from build123d import *

# Parameters (mm, degrees)
SKETCH1_R             = 9.5
SKETCH1_R_2           = 7.85
BOSS_EXTRUDE1_DEPTH   = 48
BOSS_EXTRUDE1_2_DEPTH = 48
SKETCH29_R            = 1.5
BOSS_EXTRUDE18_DEPTH  = 3
SKETCH36_R            = 1.7
BOSS_EXTRUDE26_DEPTH  = 38
SKETCH14_R            = 4.125
BOSS_EXTRUDE27_DEPTH  = 4
SKETCH34_R            = 4.2
CUT_EXTRUDE17_DEPTH   = 4.5
SKETCH38_R            = 2.15
CUT_EXTRUDE18_DEPTH   = 18.5
BOSS_EXTRUDE43_DEPTH  = 42.2
SKETCH7_R             = 1.7
BOSS_EXTRUDE44_DEPTH  = 2.8
BOSS_EXTRUDE42_START  = 25
BOSS_EXTRUDE42_DEPTH  = 6.5
BOSS_EXTRUDE45_DEPTH  = 10
SKETCH47_R            = 4
SKETCH47_R_2          = 1.5
BOSS_EXTRUDE40_DEPTH  = 1.4
CUT_EXTRUDE19_START   = -3.5
SKETCH20_R            = 1.5
SKETCH20_R_2          = 12.5
CUT_EXTRUDE19_DEPTH   = 3.5
SKETCH43_R            = 3.6
CUT_EXTRUDE22_DEPTH   = 3.5
BOSS_EXTRUDE38_DEPTH  = 4
SKETCH52_W            = 1
SKETCH52_H            = 10
BOSS_EXTRUDE36_DEPTH  = 1
SKETCH53_R            = 1.5
CUT_EXTRUDE29_DEPTH   = 4
CUT_EXTRUDE30_START   = -0.2
CUT_EXTRUDE30_DEPTH   = 0.2
CUT_EXTRUDE33_DEPTH   = 25
CUT_EXTRUDE32_DEPTH   = 8


with BuildPart() as part:
    # Sketch1 → Boss-Extrude1 (new body)
    with BuildSketch(Plane.XY):
        Circle(SKETCH1_R)
        Circle(SKETCH1_R_2, mode=Mode.SUBTRACT)
    extrude(amount=BOSS_EXTRUDE1_DEPTH)



with BuildPart() as body_2:
    # Sketch1 → Boss-Extrude1 2 (new body)
    with BuildSketch(Plane.XY):
        with Locations((52.4, 0)):
            Circle(SKETCH1_R)
        with Locations((52.4, 0)):
            Circle(SKETCH1_R_2, mode=Mode.SUBTRACT)
    extrude(amount=BOSS_EXTRUDE1_2_DEPTH)


with BuildPart() as part_1:
    add(part.part)

    add(body_2.part)  # Boss-Extrude18 merges body 2
    # Sketch29 → Boss-Extrude18 (add)
    with BuildSketch(Plane(origin=(0, 0, 0), x_dir=(-1, 0, 0), z_dir=(0, 0, -1))):
        with BuildLine():
            Line((-52.4, 9.5), (0, 9.5))
            ThreePointArc((0, 9.5), (-6.717514421, -6.717514421), (9.5, 0))
            Line((9.5, 0), (9.5, -54.1))
            ThreePointArc((9.5, -54.1), (6.717514421, -60.817514421), (0, -63.6))
            Line((0, -63.6), (-52.4, -63.6))
            ThreePointArc((-52.4, -63.6), (-59.117514421, -60.817514421), (-61.9, -54.1))
            Line((-61.9, -54.1), (-61.9, 0))
            ThreePointArc((-61.9, 0), (-53.919565268, -9.377682091), (-43.386121811, -3))
            ThreePointArc((-43.386121811, -3), (-43.093228593, -3.707106781), (-42.386121811, -4))
            Line((-42.386121811, -4), (-39.9, -4))
            ThreePointArc((-39.9, -4), (-39.192893219, -3.707106781), (-38.9, -3))
            Line((-38.9, -3), (-38.9, 3))
            ThreePointArc((-38.9, 3), (-39.192893219, 3.707106781), (-39.9, 4))
            Line((-39.9, 4), (-42.386121811, 4))
            ThreePointArc((-42.386121811, 4), (-43.093228593, 3.707106781), (-43.386121811, 3))
            ThreePointArc((-43.386121811, 3), (-46.843472307, 7.705517504), (-52.4, 9.5))
        make_face()
        with Locations(Location((-3.3, -36.55, 0), (0, 0, 180))):
            Circle(SKETCH29_R, mode=Mode.SUBTRACT)
        with Locations(Location((-17.3, -36.55, 0), (0, 0, 180))):
            Circle(SKETCH29_R, mode=Mode.SUBTRACT)
    extrude(amount=-BOSS_EXTRUDE18_DEPTH)

    # Sketch36 → Boss-Extrude26 (add)
    with BuildSketch(Plane.XY.offset(3)):
        with BuildLine():
            Line((0, 9.5), (52.4, 9.5))
            ThreePointArc((52.4, 9.5), (46.843472307, 7.705517504), (43.386121811, 3))
            ThreePointArc((43.386121811, 3), (43.093228593, 3.707106781), (42.386121811, 4))
            Line((42.386121811, 4), (39.9, 4))
            ThreePointArc((39.9, 4), (39.192893219, 3.707106781), (38.9, 3))
            Line((38.9, 3), (38.9, -3))
            ThreePointArc((38.9, -3), (39.192893219, -3.707106781), (39.9, -4))
            Line((39.9, -4), (42.386121811, -4))
            ThreePointArc((42.386121811, -4), (43.093228593, -3.707106781), (43.386121811, -3))
            ThreePointArc((43.386121811, -3), (46.843472307, -7.705517504), (52.4, -9.5))
            Line((52.4, -9.5), (0, -9.5))
            ThreePointArc((0, -9.5), (9.5, 0), (0, 9.5))
        make_face()
        with Locations(Location((25.9, 0, 0), (0, 0, 180))):
            Circle(SKETCH36_R, mode=Mode.SUBTRACT)
        with BuildLine():
            Line((31.4, 4), (32.1, 4))
            ThreePointArc((32.1, 4), (32.453553391, 3.853553391), (32.6, 3.5))
            Line((32.6, 3.5), (32.6, -3.5))
            ThreePointArc((32.6, -3.5), (32.453553391, -3.853553391), (32.1, -4))
            Line((32.1, -4), (31.4, -4))
            ThreePointArc((31.4, -4), (31.046446609, -3.853553391), (30.9, -3.5))
            Line((30.9, -3.5), (30.9, 3.5))
            ThreePointArc((30.9, 3.5), (31.046446609, 3.853553391), (31.4, 4))
        make_face(mode=Mode.SUBTRACT)
    extrude(amount=BOSS_EXTRUDE26_DEPTH)

    # Sketch14 → Boss-Extrude27 (add)
    with BuildSketch(Plane.XZ.offset(9.5)):
        with Locations(Location((14.4, 28.5, 0), (0, 0, 180))):
            Circle(SKETCH14_R)
    extrude(amount=BOSS_EXTRUDE27_DEPTH)

    # Sketch34 → Cut-Extrude17 (cut)
    with BuildSketch(Plane(origin=(0, 9.5, 0), x_dir=(1, 0, 0), z_dir=(0, 1, 0))):
        with Locations(Location((14.4, -28.5, 0), (0, 0, 180))):
            Circle(SKETCH34_R)
    extrude(amount=-CUT_EXTRUDE17_DEPTH, mode=Mode.SUBTRACT)

    # Sketch38 → Cut-Extrude18 (cut)
    with BuildSketch(Plane(origin=(0, 5, 0), x_dir=(1, 0, 0), z_dir=(0, 1, 0))):
        with Locations(Location((14.5, -28.5, 0), (0, 0, 270))):
            Circle(SKETCH38_R)
    extrude(amount=-CUT_EXTRUDE18_DEPTH, mode=Mode.SUBTRACT)

    # Sketch39 → Boss-Extrude43 (add)
    with BuildSketch(Plane.XY.offset(3)):
        with BuildLine():
            Line((41.4, -63.6), (37.9, -63.6))
            Line((37.9, -63.6), (37.9, -5))
            ThreePointArc((37.9, -5), (38.192893219, -4.292893219), (38.9, -4))
            Line((38.9, -4), (42.386121811, -4))
            ThreePointArc((42.386121811, -4), (43.093228593, -3.707106781), (43.386121811, -3))
            ThreePointArc((43.386121811, -3), (46.843472307, -7.705517504), (52.4, -9.5))
            Line((52.4, -9.5), (41.4, -9.5))
            Line((41.4, -9.5), (41.4, -63.6))
        make_face()
    extrude(amount=BOSS_EXTRUDE43_DEPTH)

    # Sketch7 → Boss-Extrude44 (add)
    with BuildSketch(Plane.XY.offset(45.2)):
        with BuildLine():
            Line((38.9, -4), (42.386121811, -4))
            ThreePointArc((42.386121811, -4), (43.093228593, -3.707106781), (43.386121811, -3))
            ThreePointArc((43.386121811, -3), (52.410945742, -9.499993694), (61.420767352, -2.979220768))
            Line((61.420767352, -2.979220768), (41.4, -63.6))
            Line((41.4, -63.6), (37.9, -63.6))
            Line((37.9, -63.6), (37.9, -5))
            ThreePointArc((37.9, -5), (38.192893219, -4.292893219), (38.9, -4))
        make_face()
        with Locations(Location((47.4, -15.6, 0), (0, 0, 180))):
            Circle(SKETCH7_R, mode=Mode.SUBTRACT)
    extrude(amount=BOSS_EXTRUDE44_DEPTH)

    # Sketch69 → Boss-Extrude42 (add)
    with BuildSketch(Plane.ZY.offset(-37.9).offset(BOSS_EXTRUDE42_START)):
        Polygon((3, -9.5), (3, -25), (18.5, -9.5), align=None)
    extrude(amount=BOSS_EXTRUDE42_DEPTH)

    # Sketch40 → Boss-Extrude45 (add)
    with BuildSketch(Plane(origin=(0, 0, 45.2), x_dir=(-1, 0, 0), z_dir=(0, 0, -1))):
        with BuildLine():
            Line((-42.2, -12.85), (-41.4, -12.85))
            Line((-41.4, -12.85), (-41.4, -18.15))
            Line((-41.4, -18.15), (-42.2, -18.15))
            ThreePointArc((-42.2, -18.15), (-42.553553391, -18.003553391), (-42.7, -17.65))
            Line((-42.7, -17.65), (-42.7, -13.35))
            ThreePointArc((-42.7, -13.35), (-42.553553391, -12.996446609), (-42.2, -12.85))
        make_face()
    extrude(amount=BOSS_EXTRUDE45_DEPTH)

    # Sketch47 → Boss-Extrude40 (add)
    with BuildSketch(Plane(origin=(41.4, 0, 0), x_dir=(0, 0, -1), z_dir=(1, 0, 0))):
        with Locations(Location((-8.5, -15.55, 0), (0, 0, 180))):
            Circle(SKETCH47_R)
        with Locations((-8.5, -15.55)):
            Circle(SKETCH47_R_2, mode=Mode.SUBTRACT)
    extrude(amount=BOSS_EXTRUDE40_DEPTH)

    # Sketch20 → Cut-Extrude19 (cut)
    with BuildSketch(Plane(origin=(41.4, 0, 0), x_dir=(0, 0, -1), z_dir=(1, 0, 0)).offset(CUT_EXTRUDE19_START)):
        with Locations((-8.5, -58.1)):
            Circle(SKETCH20_R)
        with Locations((-39.5, -58.1)):
            Circle(SKETCH20_R)
        with Locations((-8.5, -27.1)):
            Circle(SKETCH20_R)
        with Locations((-24, -42.6)):
            Circle(SKETCH20_R_2)
        with Locations(Location((-8.5, -15.55, 0), (0, 0, 90))):
            Circle(SKETCH20_R)
    extrude(amount=CUT_EXTRUDE19_DEPTH, mode=Mode.SUBTRACT)

    # Sketch43 → Cut-Extrude22 (cut)
    with BuildSketch(Plane.XY.offset(41)):
        with Locations((25.9, 0)):
            Circle(SKETCH43_R)
    extrude(amount=-CUT_EXTRUDE22_DEPTH, mode=Mode.SUBTRACT)

    # Sketch59 → Boss-Extrude38 (add)
    with BuildSketch(Plane.XY.offset(41)):
        with BuildLine():
            Line((11.2, 9.5), (41.2, 9.5))
            ThreePointArc((41.2, 9.5), (40.492893219, 9.792893219), (40.2, 10.5))
            Line((40.2, 10.5), (40.2, 47.05))
            Line((40.2, 47.05), (12.2, 47.05))
            Line((12.2, 47.05), (12.2, 10.5))
            ThreePointArc((12.2, 10.5), (11.907106781, 9.792893219), (11.2, 9.5))
        make_face()
    extrude(amount=-BOSS_EXTRUDE38_DEPTH)

    # Sketch52 → Boss-Extrude36 (add)
    with BuildSketch(Plane(origin=(-30, 0, 37), x_dir=(-1, 0, 0), z_dir=(0, 0, -1))):
        with Locations((-69.7, 42.05)):
            Rectangle(SKETCH52_W, SKETCH52_H)
        with Locations((-42.7, 42.05)):
            Rectangle(SKETCH52_W, SKETCH52_H)
    extrude(amount=BOSS_EXTRUDE36_DEPTH)

    # Sketch53 → Cut-Extrude29 (cut)
    with BuildSketch(Plane(origin=(-30, 0, 37), x_dir=(-1, 0, 0), z_dir=(0, 0, -1))):
        with Locations((-48.2, 42.05)):
            Circle(SKETCH53_R)
        with Locations((-56.2, 42.05)):
            Circle(SKETCH53_R)
        with BuildLine():
            Line((-68.2, 31.05), (-68.2, 27.05))
            ThreePointArc((-68.2, 27.05), (-67.2, 26.05), (-66.2, 27.05))
            Line((-66.2, 27.05), (-66.2, 31.05))
            ThreePointArc((-66.2, 31.05), (-67.2, 32.05), (-68.2, 31.05))
        make_face()
        with BuildLine():
            Line((-46.2, 31.05), (-46.2, 27.05))
            ThreePointArc((-46.2, 27.05), (-45.2, 26.05), (-44.2, 27.05))
            Line((-44.2, 27.05), (-44.2, 31.05))
            ThreePointArc((-44.2, 31.05), (-45.2, 32.05), (-46.2, 31.05))
        make_face()
    extrude(amount=-CUT_EXTRUDE29_DEPTH, mode=Mode.SUBTRACT)

    # Sketch62 → Cut-Extrude30 (cut)
    with BuildSketch(Plane.XY.offset(3).offset(CUT_EXTRUDE30_START)):
        with BuildLine():
            Line((61.9, -54.1), (61.9, 0))
            ThreePointArc((61.9, 0), (59.117514421, -6.717514421), (52.4, -9.5))
            Line((52.4, -9.5), (41.4, -9.5))
            Line((41.4, -9.5), (41.4, -63.6))
            Line((41.4, -63.6), (52.4, -63.6))
            ThreePointArc((52.4, -63.6), (59.117514421, -60.817514421), (61.9, -54.1))
        make_face()
    extrude(amount=CUT_EXTRUDE30_DEPTH, mode=Mode.SUBTRACT)

    # Sketch70 → Cut-Extrude33 (cut)
    with BuildSketch(Plane(origin=(0, 0, 0), x_dir=(-1, 0, 0), z_dir=(0, 0, -1))):
        with BuildLine():
            Line((-33.9, -6.5), (-22.9, -6.5))
            ThreePointArc((-22.9, -6.5), (-21.485786438, -5.914213562), (-20.9, -4.5))
            Line((-20.9, -4.5), (-20.9, 4.5))
            ThreePointArc((-20.9, 4.5), (-21.485786438, 5.914213562), (-22.9, 6.5))
            Line((-22.9, 6.5), (-33.9, 6.5))
            ThreePointArc((-33.9, 6.5), (-35.314213562, 5.914213562), (-35.9, 4.5))
            Line((-35.9, 4.5), (-35.9, -4.5))
            ThreePointArc((-35.9, -4.5), (-35.314213562, -5.914213562), (-33.9, -6.5))
        make_face()
    extrude(amount=-CUT_EXTRUDE33_DEPTH, mode=Mode.SUBTRACT)

    # Sketch66 → Cut-Extrude32 (cut)
    with BuildSketch(Plane(origin=(0, 0, 25), x_dir=(-1, 0, 0), z_dir=(0, 0, -1))):
        with BuildLine():
            Line((-31.4, 4), (-32.9, 4))
            ThreePointArc((-32.9, 4), (-33.253553391, 3.853553391), (-33.4, 3.5))
            Line((-33.4, 3.5), (-33.4, -3.5))
            ThreePointArc((-33.4, -3.5), (-33.253553391, -3.853553391), (-32.9, -4))
            Line((-32.9, -4), (-31.4, -4))
            ThreePointArc((-31.4, -4), (-31.046446609, -3.853553391), (-30.9, -3.5))
            Line((-30.9, -3.5), (-30.9, 3.5))
            ThreePointArc((-30.9, 3.5), (-31.046446609, 3.853553391), (-31.4, 4))
        make_face()
    extrude(amount=-CUT_EXTRUDE32_DEPTH, mode=Mode.SUBTRACT)


solid = part_1.part
Geometry check sheet. Reference: the model listing, model coordinates, mm. A direction names the side the tool comes from. Coordinates: 2 decimals unless noted, no trailing zeros. Order: outer loops, then holes, each group sorted by start corner. A loop starts at its lowest first (then second) coordinate and runs counter-clockwise, first axis right, second up. Notation, with made-up numbers: (20.25, 20.25) -> (48.25, 20.25) arc R24 ccw to (48.25, 34.25) -> close; hole circle Ø1 at (-13.75, -5.75). An arc over 180 degrees is marked (long way). Use a Markdown table: item, result. Add a question column.
1. Cross-section at C-C (z = 20). Give the number of separate pieces and of enclosed holes in the cut face, and give its area (3 significant figures).
2. Cross-section at A-A (z = 42.5). Enter the section's corners in (x, y), and give its area (3 significant figures).
3. Go/stop test with flat-tipped pins: pin 1 Ø10 at (y, z) = (-0.5, 15) entering from -X; pin 2 Ø4.5 at (y, z) = (-15, 12) entering from +X; pin 3 Ø2 at (x, z) = (1, 39) entering from -Y; pin 4 Ø23.5 at (x, y) = (7, -28.5) entering from +Z. Record where each tip stops, or that it passes through.
4. Mould release check, pull along Z, two halves, no side actions. Record for faces 5 (the face through (33.4, 0, 29)), 6 (the face through (47, -27, 48)), 7 (the face through (39.625, -28.564, 8.825)): pulls with the +Z half, pulls with the -Z half, needs draft (parallel to the pull), parting line crosses it, or undercut.
5. Cross-section at D-D (x = -1.5). Enter the section's corners in (y, z).
6. Cross-section at B-B (y = 42.05). Enter the section's corners in (x, z), and give its area (3 significant figures).
7. Material ranges on L1, parallel to X at y = -36.55, z = 2; L2, parallel to Y at x = 40.45, z = 8.5; L3, parallel to Y at x = 25, z = 38, recorded low to high.
8. Set-up check for faces 1 (the face through (12.14, 7.28, 32.04)), 2 (the face through (38.2, 29, 39)), 3 (the face through (42.8, -13.8, 8.4)), 4 (the face through (12.6, -13.5, 30.3)): record each of +Z, -Z, +X, -X, +Y, -Y from which the full face is reachable in a straight line by a thin tool's end or side.
Filled sheet:
| question | item | result |
|---|---|---|
| 1 | separate pieces | 2 |
| 1 | enclosed holes | 4 |
| 1 | area | 774 mm2 |
| 2 | outline | circle Ø19 at (0, 0); (37.9, -63.6) -> (41.4, -63.6) -> (41.4, -18.15) -> (42.2, -18.15) arc R0.5 ccw to (42.7, -17.65) -> (42.7, -13.35) arc R0.5 ccw to (42.2, -12.85) -> (41.4, -12.85) -> (41.4, -9.5) -> (52.4, -9.5) arc R9.5 ccw (long way) to (43.39, -3) arc R1 cw to (42.39, -4) -> (38.9, -4) arc R1 ccw to (37.9, -5) -> close; hole circle Ø15.7 at (0, 0); hole circle Ø15.7 at (52.4, 0) |
| 2 | area | 422 mm2 |
| 3 | pin 1 | x = -9.5 |
| 3 | pin 2 | x = 42.8 |
| 3 | pin 3 | y = -9.5 |
| 3 | pin 4 | z = 11.25 |
| 4 | face 5 | needs draft |
| 4 | face 6 | pulls with the +Z half |
| 4 | face 7 | undercut |
| 5 | outline | (-63.48, 0) -> (-7.71, 0) -> (-7.71, 48) -> (-9.38, 48) -> (-9.38, 3) -> (-63.48, 3) -> close; (7.71, 0) -> (9.38, 0) -> (9.38, 48) -> (7.71, 48) -> close |
| 6 | outline | (12.2, 36) -> (13.2, 36) -> (13.2, 37) -> (16.7, 37) -> (16.7, 41) -> (12.2, 41) -> close; (19.7, 37) -> (24.7, 37) -> (24.7, 41) -> (19.7, 41) -> close; (27.7, 37) -> (39.2, 37) -> (39.2, 36) -> (40.2, 36) -> (40.2, 41) -> (27.7, 41) -> close |
| 6 | area | 90.0 mm2 |
| 7 | L1 | -9.5 to 1.8, 4.8 to 15.8, 18.8 to 61.9 |
| 7 | L2 | -63.6 to -59.6, -56.6 to -28.6, -25.6 to -17.05, -14.05 to -4, 4 to 9.5 |
| 7 | L3 | -9.5 to -3.49, 3.49 to 41.15, 42.95 to 47.05 |
| 8 | face 1 | +Y |
| 8 | face 2 | +Z, -Z |
| 8 | face 3 | +X, -Y |
| 8 | face 4 | +Z, -X, -Y |
